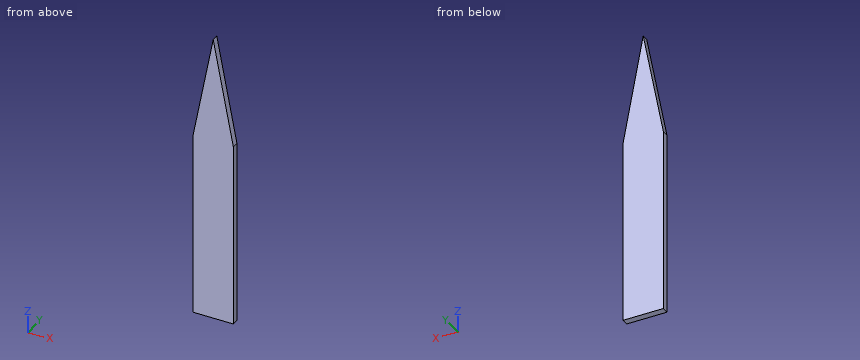
```python
from build123d import *

# Parameters (mm, degrees)
F1_DEPTH = 3.175
F3_DEPTH = 25.4


# Not quite as in the source:
# - a length typed as a fraction of an inch, garbled in the dataset ("3 / 203.2 mm" for 3/8 in), is restored


with BuildPart() as f1:
    # F0 (on Front) → F1 (new body)
    with BuildSketch(Plane.XZ):
        Polygon((0, 88.9), (0, 0), (19.05, 0), (19.05, 88.9), (9.525, 139.7), align=None)
        Polygon((0, 139.7), (0, 88.9), (9.525, 139.7), align=None)
        Polygon((9.525, 139.7), (19.05, 88.9), (19.05, 139.7), align=None)
    extrude(amount=F1_DEPTH)

    # F2 (on face) → F3 (cut)
    with BuildSketch(Plane.XZ.offset(3.175)):
        Polygon((0, 139.7), (0, 88.9), (9.525, 139.7), align=None)
        Polygon((19.05, 139.7), (9.525, 139.7), (19.05, 88.9), align=None)
    extrude(amount=-F3_DEPTH, mode=Mode.SUBTRACT)


solid = f1.part
```
Geometry check sheet. Reference: the model listing, model coordinates, mm. Give positions to 0.01 mm unless a question says otherwise; leave off trailing zeros. Write each loop counter-clockwise with the first axis right and the second up, starting at its lowest first coordinate (ties: lowest second). Pieces come first, ordered by that corner, then holes. Notation, with made-up numbers: (-15, 7) - (40, 7) arc R16 ccw to (40, 35) - close; hole circle Ø3 at (-32, -11.5). An arc over 180 degrees is marked (long way). Use a Markdown table: item, result.
Q1. Section check C-C, the plane z = 115. Enter the section's corners in (x, y) (3 decimals), then the cut area to 3 significant figures.
Computed:
| item | result |
|---|---|
| outline | (4.894, -3.175) - (14.156, -3.175) - (14.156, 0) - (4.894, 0) - close |
| area | 29.4 mm² |
Q2. Thickness scan on L1, parallel to X at y = -2.65, z = 92; L2, parallel to X at y = -2.1, z = 95.5. Record the ranges inside material, lowest first. Write a range as [from, to].
Computed:
| item | result |
|---|---|
| L1 | x = [0.58, 18.47] |
| L2 | x = [1.24, 17.81] |
Q3. Section check A-A, the plane y = -0.9. Enter the section's corners in (x, z) (3 decimals), then the cut area to 3 significant figures.
Computed:
| item | result |
|---|---|
| outline | (0, 0) - (19.05, 0) - (19.05, 88.9) - (9.525, 139.7) - (0, 88.9) - close |
| area | 2,180 mm² |
Q4. Section check B-B, the plane x = 5.25. Enter the section's corners in (y, z) (3 decimals).
Computed:
| item | result |
|---|---|
| outline | (-3.175, 0) - (0, 0) - (0, 116.9) - (-3.175, 116.9) - close |
